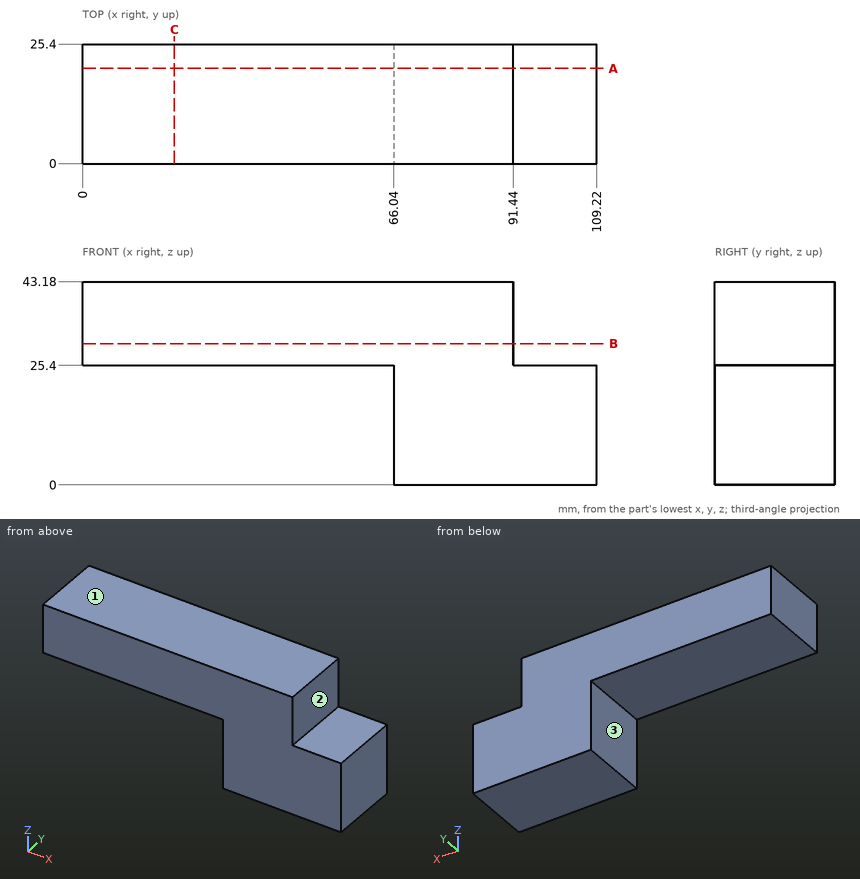
Design review of the part shown in the three views and the two pictorial views. Dimensions are in mm from the part's minimum x, y and z. A direction names the side the tool comes from. Give positions to 0.01 mm unless a question says otherwise; leave off trailing zeros. Order: outer loops, then holes, each group sorted by start corner. A loop starts at its lowest first (then second) coordinate and runs counter-clockwise, first axis right, second up. Notation, with made-up numbers: (67, -11.5) -> (91, -11.5) arc R19 cw to (91, 3.5) -> close; hole circle Ø5 at (31.5, 8). An arc over 180 degrees is marked (long way). Write each question's results on one line, items separated by ' | '. Start each with the question number.
Q1. Add section A-A on y = 20.25. Give the boundary of the cut face in (x, z), and give its area (3 significant figures).
Q2. Wall thickness on L1, parallel to X at y = 18.75, z = 11; L2, parallel to Z at x = 8, y = 10.25; L3, parallel to X at y = 8.25, z = 40: over which ranges is each line inside the solid? List them lowest first. Write a range as from..to.
Q3. For pin 1 (12.5 mm diameter, centred on x = 26, y = 14.5, fed in from -Z); pin 2 (10 mm diameter, centred on y = 6.5, z = 12, fed in from -X); pin 3 (6 mm diameter, centred on y = 8, z = 30, fed in from +X), all flat-tipped, find the tip position at first contact; note any pin that passes through.
Q4. Machinability: for the marked faces 1, 2 and 3, which of the approach directions +Z, -Z, +X, -X, +Y, -Y give a long, thin tool a straight path to every point of the face, cutting with its end or side? Answer none if there is none.
Q5. Add section C-C on x = 19.5. Give the boundary of the cut face in (y, z).
Q6. Add section B-B on z = 30. Give the boundary of the cut face in (x, y), and give its area (3 significant figures).
Found:
1) outline: (0, 25.4) -> (66.04, 25.4) -> (66.04, 0) -> (109.22, 0) -> (109.22, 25.4) -> (91.44, 25.4) -> (91.44, 43.18) -> (0, 43.18) -> close | area: 2,720 mm2
2) L1: x = 66.04..109.22 | L2: z = 25.4..43.18 | L3: x = 0..91.44
3) pin 1: stops at z = 25.4 | pin 2: stops at x = 66.04 | pin 3: stops at x = 91.44
4) face 1: +Z, +X, -X, +Y, -Y | face 2: +Z, +X, +Y, -Y | face 3: -Z, -X, +Y, -Y
5) outline: (0, 25.4) -> (25.4, 25.4) -> (25.4, 43.18) -> (0, 43.18) -> close
6) outline: (0, 0) -> (91.44, 0) -> (91.44, 25.4) -> (0, 25.4) -> close | area: 2,320 mm2
